from build123d import *

# Parameters (mm, degrees)
F2_R            = 3.0529538636
F3_DEPTH        = 15.875
F5_DEPTH        = 0.79375
F5_DEPTH_BACK   = 0.79375
F5_COPIES_COUNT = 4
F6_R            = 3.175
F7_DEPTH        = 2.921


# Not quite as in the source:
# - a pattern or mirror of a feature is missing from the dataset's text; its kind, count and spacing are read off the source's solid


with BuildPart() as f1:
    # F0 (on Top) → F1 (revolve)
    with BuildSketch(Plane.XY):
        Polygon((0, 3.175), (0, 0), (15.875, 0), (15.875, 5.08), (8.001, 5.08), (8.001, 14.9225), (2.921, 14.9225), (2.921, 3.175), align=None)
    revolve(axis=Axis((7.9375, 0, 0), (-1, 0, 0)))

    # F2 (on face) → F3 (cut, through all)
    with BuildSketch(Plane.YZ.offset(15.875)):
        Circle(F2_R)
    extrude(amount=-F3_DEPTH, mode=Mode.SUBTRACT)

    # F4 (on Front) → F5 (join, two sides)
    with BuildSketch(Plane.XZ) as f5_sk:
        Polygon((15.875, 4.1275), (8.001, 14.9225), (8.001, 4.1275), align=None)
    f5 = extrude(amount=F5_DEPTH) + extrude(f5_sk.sketch, amount=-F5_DEPTH_BACK)

    # F5_copies: F5 ×4 about axis
    f5_copies_axis = Axis((0, 0, 0), (1, 0, 0))
    for i in range(1, F5_COPIES_COUNT):
        add(f5.rotate(f5_copies_axis, i * 360 / F5_COPIES_COUNT))

    # F6 (on face) → F7 (cut, through all)
    with BuildSketch(Plane(origin=(0, 0, 0), x_dir=(0, -1, 0), z_dir=(-1, 0, 0))):
        Circle(F6_R)
    extrude(amount=-F7_DEPTH, mode=Mode.SUBTRACT)


solid = f1.part
Design review of the part built by this model. Coordinates are the model's own, in mm. A direction names the side the tool comes from. Round coordinates to 2 decimals unless told otherwise and drop trailing zeros. Write each loop counter-clockwise with the first axis right and the second up, starting at its lowest first coordinate (ties: lowest second). Pieces come first, ordered by that corner, then holes.
Item 1: Draft analysis for pull direction Y (two halves, no side actions). For faces 6 (the cylindrical face through (9.49, 2.91, 0.92)), 7 (the cylindrical face through (5.425, 14.233, -4.482)), 8 (the flat face through (10, 0.794, 8)), 9 (the flat face through (10, -8, 0.794)), state which applies: released by +Y, released by -Y, zero draft, split by the parting line, or undercut.
Item 2: Consider section D-D on z = 12.75. Give the boundary of the cut face in (x, y), and give its area (3 significant figures).
Item 3: For pin 1 Ø3.5 at (x, y) = (10.5, -11.5) entering from +Z; pin 2 Ø5 at (x, z) = (9, -9) entering from -Y; pin 3 Ø3.5 at (x, z) = (10.5, 9.5) entering from -Y, all flat-tipped, find the tip position at first contact; note any pin that passes through.
Item 4: For faces 1 (the flat face through (10, -8, -0.794)), 2 (the flat face through (10, -0.794, 8)), 3 (the flat face through (11.664, -0.011, 9.901)), 4 (the flat face through (10, 8, 0.794)), 5 (the flat face through (8.001, 6, -6)), list the 3-axis set-ups (+Z, -Z, +X, -X, +Y, -Y) from which the entire face can be reached by the end or side of a thin tool; tool diameter is ignored.
Item 5: Consider section A-A on x = 9.75. Give the boundary of the cut face in (y, z), and give its area (3 significant figures).
Item 6: Consider section B-B on z = -1.5. Give the boundary of the cut face in (x, y) (1 decimal).
Item 7: Consider section C-C on y = 9.25. Give the boundary of the cut face in (x, z), and give its area (3 significant figures).
Item 8: Wall thickness on L1, parallel to Z at x = 6, y = 0; L2, parallel to Z at x = 10.5, y = -7.5; L3, parallel to X at y = -4.5, z = 8.5: over which ranges is each line inside the solid? List them lowest first.
Check values:
1. face 6: undercut
1. face 7: split by the parting line
1. face 8: released by +Y
1. face 9: zero draft
2. outline: (2.92, -7.75) - (8, -7.75) - (8, -0.79) - (9.59, -0.79) - (9.59, 0.79) - (8, 0.79) - (8, 7.75) - (2.92, 7.75) - close
2. area: 81.3 mm2
3. pin 1: stops at z = 0.79
3. pin 2: stops at y = -13.33
3. pin 3: stops at y = -0.79
4. face 1: -Z, +X, -Y
4. face 2: +Z, +X, -Y
4. face 3: +Z, +X, +Y, -Y
4. face 4: +Z, +X, +Y
4. face 5: -Z, +X, +Y
5. outline: (-12.52, -0.79) - (-5.02, -0.79) arc R5.08 ccw to (-0.79, -5.02) - (-0.79, -12.52) - (0.79, -12.52) - (0.79, -5.02) arc R5.08 ccw to (5.02, -0.79) - (12.52, -0.79) - (12.52, 0.79) - (5.02, 0.79) arc R5.08 ccw to (0.79, 5.02) - (0.79, 12.52) - (-0.79, 12.52) - (-0.79, 5.02) arc R5.08 ccw to (-5.02, 0.79) - (-12.52, 0.79) - close; hole circle Ø6.11 at (0, 0)
5. area: 99.2 mm2
6. outline: (2.9, -14.8) - (8, -14.8) - (8, -4.9) - (15.9, -4.9) - (15.9, -2.7) - (2.9, -2.7) - close; (2.9, 2.7) - (15.9, 2.7) - (15.9, 4.9) - (8, 4.9) - (8, 14.8) - (2.9, 14.8) - close
7. outline: (2.92, -11.71) - (8, -11.71) - (8, -0.79) - (12.14, -0.79) - (12.14, 0.79) - (8, 0.79) - (8, 11.71) - (2.92, 11.71) - close
7. area: 126 mm2
8. L1: z = -14.92 to -3.05, 3.05 to 14.92
8. L2: z = -0.79 to 0.79
8. L3: x = 2.92 to 8
